Could you check a few things on this model? Use its own coordinates, in mm. A direction names the side the tool comes from. Coordinates: 2 decimals unless noted, no trailing zeros. Loops run counter-clockwise (first coordinate to the right, second up) from the corner with the lowest first, then second, coordinate; pieces in that order, holes last. Notation, with made-up numbers: (81, 11) - (134, 11) arc R23 ccw to (134, 47) - close; hole circle Ø10 at (-15, 76). An arc over 180 degrees is marked (long way). One line per item, written item: value. Start each with the question number.
(1) If we section it at B-B on y = 266: Write out the boundary of the cut face in (x, z) (3 decimals), then the cut area to 3 significant figures.
(2) If we mould it in two halves opening along Z, with no side actions, what happens to faces 5 (the face through (1152, 257.606, 62)), 6 (the face through (1084, 224, 54.564)), 7 (the face through (1018.2, 280.49, 55.71)), 8 (the face through (1152, 271, 59.604))? For each: pulls with the +Z half, pulls with the -Z half, needs draft (parallel to the pull), parting line crosses it, or undercut.
(3) I'm going to push flat-ended pins straight in: P1, Ø0.9, axis at x = 1152.5, z = 62, coming from the +Y side; P2, Ø6, axis at x = 1083.5, y = 230.5, coming from the -Z side; P3, Ø1.6, axis at x = 1152, y = 273.5, coming from the +Z side; P4, Ø0.9, axis at x = 1151.5, y = 233, coming from the -Z side. Where does each tip first touch, or does it pass through?
(4) If I drill on line 1 along X through (y, z) = (241, 63.25) (3 decimals); line 2 along Y through (x, z) = (1060.5, 57), over which ranges is the centre line in solid material (lowest first)? Write a range as from..to.
(5) On a 3-axis mill with a long thin cutter (end or side, diameter ignored), from which of +Z, -Z, +X, -X, +Y, -Y can I reach the whole of each face in a straight line? I mean faces 1 (the face through (1152, 240, 59.604)), 2 (the face through (1018, 271, 59.604)), 3 (the face through (1151.758, 274.444, 56.859)), 4 (the face through (1084, 224, 59.604)). Say none if no direction works.
(6) If we section it at A-A on y = 228: Write out the boundary of the cut face in (x, z) (3 decimals).
(7) If we section it at C-C on x = 1026.5: Write out the boundary of the cut face in (y, z), then the cut area to 3 significant figures.
```python
from build123d import *

# Parameters (mm, degrees)
SALIENTE_EXTRUIR1_DEPTH = 80
CROQUIS2_R              = 27.5
CORTAR_EXTRUIR2_DEPTH   = 2387.503718832
SALIENTE_EXTRUIR2_DEPTH = 50
CROQUIS4_W              = 80
CROQUIS4_H              = 440
CORTAR_EXTRUIR3_DEPTH   = 2390.874473691
SALIENTE_EXTRUIR3_DEPTH = 50
ESCALA1_SCALE           = 0.063
CROQUIS9_W              = 136.71
CROQUIS9_H              = 5.04
SALIENTE_EXTRUIR5_DEPTH = 13
CROQUIS10_W             = 130.41
CROQUIS10_H             = 8
CORTAR_EXTRUIR4_DEPTH   = 10
CROQUIS11_W             = 136.71
CROQUIS11_H             = 13.15
CORTAR_EXTRUIR5_DEPTH   = 1192.165803699


with BuildPart() as part:
    # Croquis1 → Saliente-Extruir1 (new body)
    with BuildSketch(Plane.XY):
        Polygon((0, 0), (2170, 0), (2170, 990), (2120, 990), (2120, 50), (50, 50), (50, 990), (0, 990), align=None)
    extrude(amount=SALIENTE_EXTRUIR1_DEPTH)

    # Croquis2 → Cortar-Extruir2 (cut, through all)
    with BuildSketch(Plane.ZY):
        with Locations((40, 940)):
            Circle(CROQUIS2_R)
        with Locations((40, 800)):
            Circle(CROQUIS2_R)
    extrude(amount=-CORTAR_EXTRUIR2_DEPTH, mode=Mode.SUBTRACT)

    # Croquis3 → Saliente-Extruir2 (add)
    with BuildSketch(Plane.ZY):
        Polygon((150, 560), (80, 560), (0, 560), (0, 500), (80, 500), (80, 60), (0, 60), (0, 0), (150, 0), align=None)
    extrude(amount=-SALIENTE_EXTRUIR2_DEPTH)

    # Croquis4 → Cortar-Extruir3 (cut, through all)
    with BuildSketch(Plane.ZY):
        with Locations((40, 280)):
            Rectangle(CROQUIS4_W, CROQUIS4_H)
    extrude(amount=-CORTAR_EXTRUIR3_DEPTH, mode=Mode.SUBTRACT)


with BuildPart() as cortar_extruir3_piece_1:
    # of the separate pieces the step leaves, piece 1, a body of its own (cortar_extruir3_pieces)
    add(part.part.solids().sort_by_distance((0, 0, 0))[0])



with BuildPart() as cortar_extruir3_piece_2:
    # of the separate pieces the step leaves, piece 2, a body of its own (cortar_extruir3_pieces)
    add(part.part.solids().sort_by_distance((2120, 500, 0))[0])


with BuildPart() as cortar_extruir3_piece_1_1:
    add(cortar_extruir3_piece_1.part)

    add(cortar_extruir3_piece_2.part)  # Saliente-Extruir3 merges Cortar-Extruir3 piece 2
    # Croquis5 → Saliente-Extruir3 (add)
    with BuildSketch(Plane(origin=(2170, 0, 0), x_dir=(0, 0, -1), z_dir=(1, 0, 0))):
        Polygon((-150, 50), (-150, 0), (0, 0), (0, 60), (-80, 60), (-80, 500), (0, 500), (0, 560), (-150, 560), align=None)
    extrude(amount=-SALIENTE_EXTRUIR3_DEPTH)


with BuildPart() as cortar_extruir3_piece_1_2:
    # Escala1: scaled about (1085, 237.274110873, 58.232745712)
    add(cortar_extruir3_piece_1_1.part.scale(ESCALA1_SCALE).moved(Location((1016.645, 222.325841888, 54.564082732))))

    # Croquis9 → Saliente-Extruir5 (add)
    with BuildSketch(Plane(origin=(0, 284.695841888, 0), x_dir=(1, 0, 0), z_dir=(0, 1, 0))):
        with Locations((1085, -57.084082732)):
            Rectangle(CROQUIS9_W, CROQUIS9_H)
    extrude(amount=SALIENTE_EXTRUIR5_DEPTH)

    # Croquis10 → Cortar-Extruir4 (cut)
    with BuildSketch(Plane.XY.offset(59.604082732)):
        with Locations((1085, 288.695841888)):
            Rectangle(CROQUIS10_W, CROQUIS10_H)
    extrude(amount=-CORTAR_EXTRUIR4_DEPTH, mode=Mode.SUBTRACT)

    # Croquis11 → Cortar-Extruir5 (cut, through all)
    with BuildSketch(Plane.XY.offset(59.604082732)):
        with Locations((1085, 291.120841888)):
            Rectangle(CROQUIS11_W, CROQUIS11_H)
    extrude(amount=-CORTAR_EXTRUIR5_DEPTH, mode=Mode.SUBTRACT)


solid = cortar_extruir3_piece_1_2.part
```
Values:
1. outline: (1016.645, 54.564) - (1019.795, 54.564) - (1019.795, 59.604) - (1016.645, 59.604) - close; (1150.205, 54.564) - (1153.355, 54.564) - (1153.355, 59.604) - (1150.205, 59.604) - close
1. area: 31.8 mm2
2. face 5: needs draft
2. face 6: pulls with the -Z half
2. face 7: undercut
2. face 8: pulls with the +Z half
3. P1: stops at y = 257.61
3. P2: passes through
3. P3: stops at z = 59.6
3. P4: stops at z = 59.6
4. line 1: x = 1016.645..1019.795, 1150.205..1153.355
4. line 2: y = 222.33..225.48
5. face 1: -Z, +X, -X
5. face 2: +Z, +X, -X, +Y
5. face 3: +X, -X
5. face 4: +Z, +Y, -Y
6. outline: (1016.645, 59.604) - (1019.795, 59.604) - (1019.795, 64.014) - (1016.645, 64.014) - close; (1150.205, 59.604) - (1153.355, 59.604) - (1153.355, 64.014) - (1150.205, 64.014) - close
7. outline: (222.33, 54.56) - (225.48, 54.56) - (225.48, 59.6) - (222.33, 59.6) - close
7. area: 15.9 mm2
